Geometry: see drawing. Coordinates: mm, zero at the bounding-box minimum. A direction names the side the tool comes from. Round coordinates to 2 decimals unless told otherwise and drop trailing zeros. Loops run counter-clockwise (first coordinate to the right, second up) from the corner with the lowest first, then second, coordinate; pieces in that order, holes last. Notation, with made-up numbers: (-20.75, 57) -> (28.25, 57) arc R5 ccw to (28.25, 65) -> close; hole circle Ø11 at (-9, -23.75). An arc over 180 degrees is marked (long way). Answer in a Markdown table with one row per item.
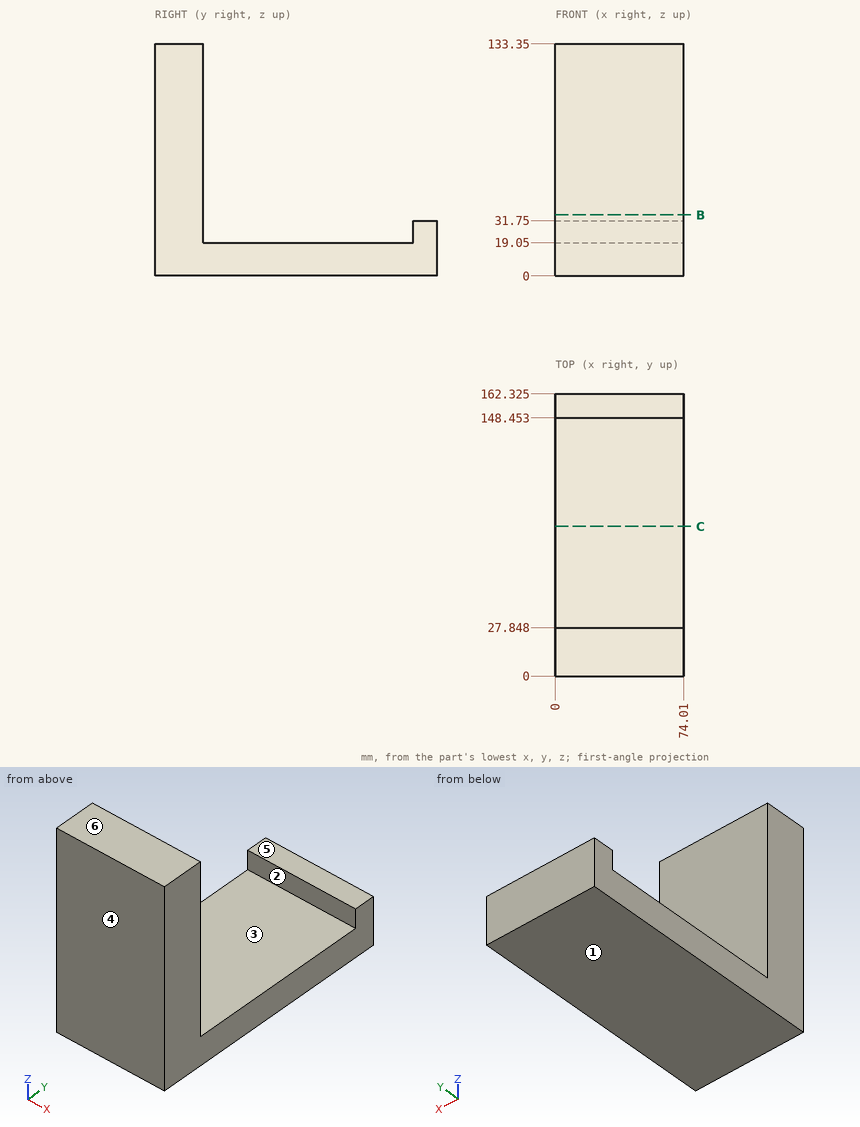
Item 1: Ray query, L1, parallel to Y at x = 29.5, z = 28 (1 decimal); L2, parallel to Y at x = 43, z = 59; L3, parallel to Z at x = 7, y = 61. Return the intervals inside material, ascending.
Ans:
| item | result |
|---|---|
| L1 | 0 to 27.8, 148.5 to 162.3 |
| L2 | 0 to 27.85 |
| L3 | 0 to 19.05 |
Item 2: Set-up query: the marked faces 5 and 6. Return all of +Z, -Z, +X, -X, +Y, -Y with unobstructed straight access to the full face (end or side cutting, diameter ignored); none if empty.
Ans:
| item | result |
|---|---|
| face 5 | +Z, +X, -X, +Y |
| face 6 | +Z, +X, -X, +Y, -Y |
Item 3: Mould query, pull axis Y, two halves, no side actions, for the marked faces 1, 2, 3 and 4. Classes: released by +Y, released by -Y, zero draft, split by the parting line, or undercut.
Ans:
| item | result |
|---|---|
| face 1 | zero draft |
| face 2 | undercut |
| face 3 | undercut |
| face 4 | released by -Y |
Item 4: Section query B-B, the plane z = 35. Output: boundary loops of the cut face in (x, y).
Ans:
| item | result |
|---|---|
| outline | (0, 0) -> (74.01, 0) -> (74.01, 27.85) -> (0, 27.85) -> close |
Item 5: First-contact query: P1, Ø10, axis at x = 59.5, y = 68, coming from the +Z side; P2, Ø6, axis at x = 39, y = 144, coming from the -Z side; P3, Ø12, axis at x = 47.5, z = 86, coming from the +Y side; P4, Ø4, axis at x = 55.5, y = 153, coming from the +Z side. Flat tips, straight axial feed; report the tip coordinate or a pass-through.
Ans:
| item | result |
|---|---|
| P1 | z = 19.05 |
| P2 | z = 0 |
| P3 | y = 27.85 |
| P4 | z = 31.75 |
Item 6: Section query C-C, the plane y = 86. Output: boundary loops of the cut face in (x, z), and give its area (3 significant figures).
Ans:
| item | result |
|---|---|
| outline | (0, 0) -> (74.01, 0) -> (74.01, 19.05) -> (0, 19.05) -> close |
| area | 1,410 mm2 |
